Autodesk Inventor part; units mm, degrees
ref_plane "YZ Plane" through (0, 0, 0) normal (1, 0, 0) x (0, 1, 0)
ref_plane "XZ Plane" through (0, 0, 0) normal (0, 1, 0) x (-1, 0, 0)
ref_plane "XY Plane" through (0, 0, 0) normal (0, 0, 1) x (1, 0, 0)
sketch "Sketch1" plane through (0, 0, 0) normal (0, 0, 1) x (1, 0, 0)
  line L0 (0, 0) -> (58, 0)
  line L1 (58, 0) -> (58, 138)
  line L2 (58, 138) -> (0, 138)
  line L3 (0, 138) -> (0, 0)
  dimension "d0" = 58
  dimension "d1" = 138
extrude "Extrusion1" add sketch "Sketch1" along normal blind 40
fillet "Fillet1" radius 10 2 edges at (0, 69, 0) (58, 69, 0)
shell "Shell1" thickness 3 removed faces 1 at (19.3333, 92, 40)
sketch "Sketch2" plane through (0, 0, 40) normal (0, 0, 1) x (1, 0, 0)
  line L0 (55, 135) -> (55, 3)
  line L1 (55, 135) -> (55, 130)
  line L2 (55, 130) -> (50, 130)
  circle A0 centre (50, 130) radius 5
  point P0 (0, 0)
  dimension "d6" = 5
  dimension "d7" = 5
extrude "Extrusion3" add sketch "Sketch2" against normal blind 10
sketch "Sketch10" plane through (0, 0, 40) normal (0, 0, 1) x (1, 0, 0)
  line L0 (3, 135) -> (50, 135)
  line L1 (48, 135) -> (55, 135)
  line L2 (50, 135) -> (55, 135)
  arc A0 (55, 130) -> (50, 135) centre (50, 130) ccw
  line L3 (55, 135) -> (50, 135)
  line L4 (55, 135) -> (55, 3)
  line L5 (55, 135) -> (55, 130)
  point P0 (0, 0)
extrude "Extrusion4" add sketch "Sketch10" against normal blind 10
sketch "Sketch11" plane through (0, 0, 40) normal (0, 0, 1) x (1, 0, 0)
  arc A0 (55, 130) -> (50, 135) centre (50, 130) ccw
  circle A1 centre (50, 130) radius 1.5
  point P0 (0, 0)
  dimension "d14" = 3
extrude "Extrusion5" cut sketch "Sketch11" against normal blind 5
thread "Thread1"
sketch "Sketch12" plane through (0, 0, 40) normal (0, 0, 1) x (1, 0, 0)
  line L0 (3, 3) -> (3, 135)
  line L1 (55, 3) -> (3, 3)
  line L2 (3, 3) -> (3, 8)
  line L3 (3, 8) -> (8, 8)
  line L4 (10, 138) -> (10, 0)
  circle A0 centre (8, 8) radius 5
  point P0 (0, 0)
  dimension "d20" = 5
  dimension "d21" = 5
extrude "Extrusion6" add sketch "Sketch12" against normal blind 10 contours A0 L4 | A0 L4
sketch "Sketch15" plane through (0, 0, 40) normal (0, 0, 1) x (1, 0, 0)
  line L0 (8, 3) -> (3, 3)
  line L1 (3, 3) -> (3, 135)
  line L2 (8, 3) -> (3, 3)
  arc A0 (3, 8) -> (8, 3) centre (8, 8) ccw
  line L3 (3, 3) -> (8, 3)
  point P0 (0, 0)
extrude "Extrusion7" add sketch "Sketch15" against normal blind 10
sketch "Sketch16" plane through (0, 0, 40) normal (0, 0, 1) x (1, 0, 0)
  arc A0 (8, 3) -> (3, 8) centre (8, 8) ccw
  circle A1 centre (8, 8) radius 1.5
  point P0 (0, 0)
  dimension "d26" = 3
extrude "Extrusion8" cut sketch "Sketch16" against normal blind 5
thread "Thread2"
sketch "Sketch17" plane through (0, 0, 40) normal (0, 0, 1) x (1, 0, 0)
  line L0 (10, 138) -> (10, 0)
  line L1 (8, 135) -> (8, 130)
  circle A0 centre (8, 130) radius 5
  point P0 (0, 0)
  point P1 (3, 135)
  dimension "d31" = 5
  dimension "d32" = 5
extrude "Extrusion9" add sketch "Sketch17" against normal blind 10
sketch "Sketch18" plane through (0, 0, 40) normal (0, 0, 1) x (1, 0, 0)
  arc A0 (8, 135) -> (3, 130) centre (8, 130) ccw
  line L0 (3, 3) -> (3, 135)
  line L1 (8, 135) -> (3, 135)
  line L2 (3, 135) -> (8, 135)
  line L3 (3, 135) -> (10, 135)
  point P0 (0, 0)
extrude "Extrusion10" add sketch "Sketch18" against normal blind 10
sketch "Sketch19" plane through (0, 0, 40) normal (0, 0, 1) x (1, 0, 0)
  arc A0 (3, 130) -> (8, 135) centre (8, 130) ccw
  circle A1 centre (8, 130) radius 1.5
  point P0 (0, 0)
  dimension "d37" = 3
extrude "Extrusion11" cut sketch "Sketch19" against normal blind 5
thread "Thread3"
sketch "Sketch21" plane through (0, 0, 40) normal (0, 0, 1) x (1, 0, 0)
  circle A0 centre (50, 8) radius 5
  point P0 (0, 0)
  point P1 (55, 3)
extrude "Extrusion12" add sketch "Sketch21" against normal blind 10
sketch "Sketch23" plane through (0, 0, 40) normal (0, 0, 1) x (1, 0, 0)
  arc A0 (50, 3) -> (55, 8) centre (50, 8) ccw
  line L0 (55, 135) -> (55, 3)
  line L1 (50, 3) -> (55, 3)
  line L2 (55, 3) -> (50, 3)
  line L3 (55, 3) -> (50, 3)
  point P0 (0, 0)
extrude "Extrusion13" add sketch "Sketch23" against normal blind 10
sketch "Sketch24" plane through (0, 0, 40) normal (0, 0, 1) x (1, 0, 0)
  arc A0 (55, 8) -> (50, 3) centre (50, 8) ccw
  circle A1 centre (50, 8) radius 1.5
  point P0 (0, 0)
  dimension "d48" = 3
extrude "Extrusion14" cut sketch "Sketch24" against normal blind 5
thread "Thread4"
sketch "Sketch25" plane through (0, 0, 40) normal (0, 0, 1) x (1, 0, 0)
  point P0 (0, 0)
properties part number "ICE CREAM"
The model under review builds one solid part; all positions refer to its coordinate system, in mm. A direction names the side the tool comes from. Give positions to 0.01 mm unless a question says otherwise; leave off trailing zeros. Write each loop counter-clockwise with the first axis right and the second up, starting at its lowest first coordinate (ties: lowest second). Pieces come first, ordered by that corner, then holes. Notation, with made-up numbers: M 2,52.5 L 29,52.5 A28 cw 29,80.5 Z; hole C 28.5,-26 d11. An arc over 180 degrees is marked long. One line per question, with ' | ' between items. Start each with the question number.
Item 1: We need section B-B on z = 26. Write out the cut boundary in (x, y), plus the area to 3 significant figures.
Item 2: Wall thickness on line 1 (X direction, y = 86, z = 19); line 2 (Y direction, x = 36.5, z = 16.5); line 3 (Z direction, x = 46, y = 53.5): over which ranges is each line inside the solid? List them lowest first. Write a range as from..to.
Item 3: We need section A-A on y = 58. Write out the cut boundary in (x, z).
Item 4: We need section D-D on z = 37. Write out the cut boundary in (x, y).
Item 5: For pin 1 (8 mm diameter, centred on x = 52.5, y = 9, fed in from -Z); pin 2 (2.5 mm diameter, centred on x = 8, y = 130, fed in from +Z); pin 3 (5 mm diameter, centred on x = 50.5, y = 97.5, fed in from +Z), all flat-tipped, find the tip position at first contact; note any pin that passes through.
Item 6: For faces 1 (the flat face through (29, 0, 20)), 2 (the flat face through (29, 3, 21)), 3 (the flat face through (50, 130, 35)), list the 3-axis set-ups (+Z, -Z, +X, -X, +Y, -Y) from which the entire face can be reached by the end or side of a thin tool; tool diameter is ignored.
Item 7: Draft analysis for pull direction Z (two halves, no side actions). For faces 4 (the flat face through (29, 70, 0)), 5 (the flat face through (50, 8, 35)), 6 (the flat face through (50, 8, 30)), state which applies: released by +Z, released by -Z, zero draft, split by the parting line, or undercut.
Item 8: We need section C-C on x = 41.5. Write out the cut boundary in (y, z).
Results found:
1) outline: M 0,0 L 58,0 L 58,138 L 0,138 Z; hole M 3,3 L 55,3 L 55,135 L 3,135 Z | area: 1,140 mm2
2) line 1: x = 0..3, 55..58 | line 2: y = 0..3, 135..138 | line 3: z = 0..3
3) outline: M 0,10 A10 ccw 10,0 L 48,0 A10 ccw 58,10 L 58,40 L 55,40 L 55,10 A7 cw 48,3 L 10,3 A7 cw 3,10 L 3,40 L 0,40 Z
4) outline: M 0,0 L 58,0 L 58,138 L 0,138 Z; hole M 3,8 A5 cw long 8,3 L 50,3 A5 cw long 55,8 L 55,130 A5 cw long 50,135 L 8,135 A5 cw long 3,130 Z; hole C 8,8 d3; hole C 8,130 d3; hole C 50,8 d3; hole C 50,130 d3
5) pin 1: stops at z = 0.01 | pin 2: stops at z = 35 | pin 3: stops at z = 5.1
6) face 1: +Z, -Z, +X, -X, -Y | face 2: none | face 3: +Z
7) face 4: released by -Z | face 5: released by +Z | face 6: undercut
8) outline: M 0,0 L 138,0 L 138,40 L 135,40 L 135,3 L 3,3 L 3,40 L 0,40 Z
